Part model, mm, in its own coordinate system. Give positions to 0.01 mm unless a question says otherwise; leave off trailing zeros. Loops run counter-clockwise (first coordinate to the right, second up) from the corner with the lowest first, then second, coordinate; pieces in that order, holes last. Notation, with made-up numbers: (84.25, -14) -> (136.25, -14) arc R33 ccw to (136.25, 18) -> close; hole circle Ø5 at (19.25, 86). An arc over 180 degrees is marked (long way). One line per question, with ' | ' between items.
```python
from build123d import *

# Parameters (mm, degrees)
SKETCH1_R           = 1.5
SKETCH1_R_2         = 3
BOSS_EXTRUDE1_DEPTH = 4


with BuildPart() as part:
    # Sketch1 → Boss-Extrude1 (new body)
    with BuildSketch(Plane.XY):
        Polygon((16.544913582, 45.848229773), (181.544913582, 45.848229773), (181.544913582, 27.848229773), (205.044913582, 27.848229773), (205.044913582, -12.151770227), (181.544913582, -12.151770227), (181.544913582, -30.151770227), (16.544913582, -30.151770227), (16.544913582, -12.151770227), (-6.955086418, -12.151770227), (-6.955086418, 27.848229773), (16.544913582, 27.848229773), align=None)
        with Locations((21.544913582, -25.151770227)):
            Circle(SKETCH1_R, mode=Mode.SUBTRACT)
        with Locations(Location((176.544913582, -25.151770227, 0), (0, 0, 180))):
            Circle(SKETCH1_R, mode=Mode.SUBTRACT)
        with Locations((176.544913582, 40.848229773)):
            Circle(SKETCH1_R, mode=Mode.SUBTRACT)
        with Locations(Location((21.544913582, 40.848229773, 0), (0, 0, 180))):
            Circle(SKETCH1_R, mode=Mode.SUBTRACT)
        with Locations((199.044913582, 7.848229773)):
            Circle(SKETCH1_R_2, mode=Mode.SUBTRACT)
        with Locations(Location((-0.955086418, 7.848229773, 0), (0, 0, 180))):
            Circle(SKETCH1_R_2, mode=Mode.SUBTRACT)
    extrude(amount=BOSS_EXTRUDE1_DEPTH)


solid = part.part
```
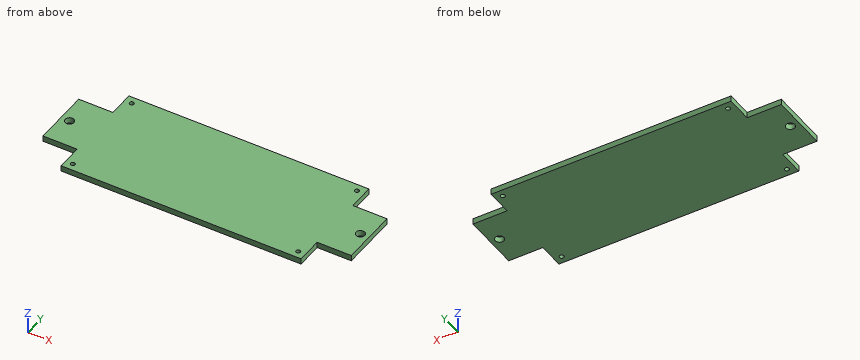
1) Saw through at A-A (z = 2.1). Give the cut face in (x, y), and give its area (3 significant figures).
Found:
outline: (-6.96, -12.15) -> (16.54, -12.15) -> (16.54, -30.15) -> (181.54, -30.15) -> (181.54, -12.15) -> (205.04, -12.15) -> (205.04, 27.85) -> (181.54, 27.85) -> (181.54, 45.85) -> (16.54, 45.85) -> (16.54, 27.85) -> (-6.96, 27.85) -> close; hole circle Ø6 at (-0.96, 7.85); hole circle Ø3 at (21.54, -25.15); hole circle Ø3 at (21.54, 40.85); hole circle Ø3 at (176.54, -25.15); hole circle Ø3 at (176.54, 40.85); hole circle Ø6 at (199.04, 7.85) | area: 14,300 mm2
2) Pin check, flat tips, straight feed: P1, Ø2, axis at y = 34.5, z = 2.5, coming from the +X side; P2, Ø1.2, axis at y = 37.5, z = 2, coming from the -X side; P3, Ø2, axis at x = 8.5, z = 2.5, coming from the -Y side; P4, Ø2.5, axis at x = 21.54, y = 40.85, coming from the +Z side. Stop position of each tip, or through.
Found:
P1: x = 181.54 | P2: x = 16.54 | P3: y = -12.15 | P4: through
3) Saw through at C-C (x = 6.5). Give the cut face in (y, z).
Found:
outline: (-12.15, 0) -> (27.85, 0) -> (27.85, 4) -> (-12.15, 4) -> close
4) Drill centre lines: line 1 (X direction, y = 8, z = 2.3); line 2 (Y direction, x = 22.5, z = 1.5); line 3 (X direction, y = -21.5, z = 1.2). Where is each one in solid material? Low to high.
Found:
line 1: -6.96 to -3.95, 2.04 to 196.05, 202.04 to 205.04 | line 2: -30.15 to -26.31, -24 to 39.69, 42 to 45.85 | line 3: 16.54 to 181.54
5) Saw through at B-B (y = 31). Give the cut face in (x, z), and give its area (3 significant figures).
Found:
outline: (16.54, 0) -> (181.54, 0) -> (181.54, 4) -> (16.54, 4) -> close | area: 660 mm2
